```python
from build123d import *

# Parameters (mm, degrees)
SKETCH1_W      = 203.2
SKETCH1_H      = 101.6
EXTRUDE1_DEPTH = 50.8
EXTRUDE2_DEPTH = 16.51
SKETCH20_W     = 203.2
SKETCH20_H     = 50.8
EXTRUDE3_DEPTH = 1270


with BuildPart() as part:
    # Sketch1 → Extrude1 (new body)
    with BuildSketch(Plane.XY):
        with Locations((101.6, 50.8)):
            Rectangle(SKETCH1_W, SKETCH1_H)
    extrude(amount=EXTRUDE1_DEPTH)

    # Sketch6 → Extrude2 (add)
    with BuildSketch(Plane.XY.offset(50.8)):
        with BuildLine():
            ThreePointArc((37.627484075, 52.10066287), (41.730641244, 51.143940803), (45.529464649, 52.96607049))
            Line((45.529464649, 52.96607049), (64.421207315, 71.857813157))
            ThreePointArc((64.421207315, 71.857813157), (66.159065786, 75.109117673), (65.797714286, 78.777981013))
            Line((65.797714286, 78.777981013), (63.063921217, 85.377941317))
            Line((63.063921217, 85.377941317), (69.784164904, 91.197771623))
            Line((69.784164904, 91.197771623), (72.499996333, 84.641174554))
            Line((72.499996333, 84.641174554), (79.539958371, 87.557222308))
            Line((79.539958371, 87.557222308), (81.969998167, 81.690587277))
            Line((81.969998167, 81.690587277), (74.930036129, 78.774539522))
            Line((74.930036129, 78.774539522), (77.56029225, 72.424539522))
            Line((77.56029225, 72.424539522), (43.43531899, 38.299566262))
            Line((43.43531899, 38.299566262), (34.866461901, 43.758530283))
            Line((34.866461901, 43.758530283), (37.302310042, 45.218374053))
            Line((37.302310042, 45.218374053), (31.946774361, 48.630226566))
            Line((31.946774361, 48.630226566), (31.653140492, 45.805641791))
            Line((31.653140492, 45.805641791), (23.4233337, 51.04860695))
            Line((23.4233337, 51.04860695), (30.143577387, 56.868437256))
            Line((30.143577387, 56.868437256), (37.627484075, 52.10066287))
        make_face()
        Polygon((31.946774361, 48.630226566), (31.653140492, 45.805641791), (27.558917476, 39.378998974), (30.772238885, 37.331887466), (34.866461901, 43.758530283), (37.302310042, 45.218374053), align=None)
    extrude(amount=EXTRUDE2_DEPTH)

    # Sketch20 → Extrude3 (cut)
    with BuildSketch(Plane.XZ):
        with Locations((101.6, 25.4)):
            Rectangle(SKETCH20_W, SKETCH20_H)
    extrude(amount=-EXTRUDE3_DEPTH, mode=Mode.SUBTRACT)


solid = part.part
```
Part model, mm, in its own coordinate system. A direction names the side the tool comes from. Round coordinates to 2 decimals unless told otherwise and drop trailing zeros. Loops run counter-clockwise (first coordinate to the right, second up) from the corner with the lowest first, then second, coordinate; pieces in that order, holes last. Notation, with made-up numbers: (66, 20.5) -> (73, 20.5) arc R16 cw to (73, 38.5) -> close; hole circle Ø11 at (0.25, 66). An arc over 180 degrees is marked (long way). Use a Markdown table: item, result.
1) Cut at A-A, the plane x = 29. List the corners of the cut face in (y, z), and give its area (3 significant figures).
The answers:
| item | result |
|---|---|
| outline | (38.46, 50.8) -> (41.64, 50.8) -> (41.64, 67.31) -> (38.46, 67.31) -> close; (47.5, 50.8) -> (55.88, 50.8) -> (55.88, 67.31) -> (47.5, 67.31) -> close |
| area | 191 mm2 |
2) Cut at D-D, the plane x = 69. List the corners of the cut face in (y, z), and give its area (3 significant figures).
The answers:
| item | result |
|---|---|
| outline | (63.86, 50.8) -> (90.52, 50.8) -> (90.52, 67.31) -> (63.86, 67.31) -> close |
| area | 440 mm2 |
3) Cut at B-B, the plane z = 64.5. List the corners of the cut face in (x, y), and give its area (3 significant figures).
The answers:
| item | result |
|---|---|
| outline | (23.42, 51.05) -> (31.65, 45.81) -> (27.56, 39.38) -> (30.77, 37.33) -> (34.87, 43.76) -> (43.44, 38.3) -> (77.56, 72.42) -> (74.93, 78.77) -> (81.97, 81.69) -> (79.54, 87.56) -> (72.5, 84.64) -> (69.78, 91.2) -> (63.06, 85.38) -> (65.8, 78.78) arc R6.35 cw to (64.42, 71.86) -> (45.53, 52.97) arc R6.35 cw to (37.63, 52.1) -> (30.14, 56.87) -> close |
| area | 755 mm2 |
4) Tool access for faces 5 (the flat face through (32.79, 40.5, 58.94)), 6 (the flat face through (76.23, 75.64, 58.94)), 7 (the flat face through (27.6, 48.39, 58.94)), 8 (the flat face through (26.74, 53.92, 58.94)), 9 (the flat face through (71.12, 87.97, 58.94)): list every direction of +Z, -Z, +X, -X, +Y, -Y with a clear straight run to the whole face (end or side of a thin tool).
The answers:
| item | result |
|---|---|
| face 5 | +Z, -Z, -Y |
| face 6 | +Z, -Z, +X |
| face 7 | +Z, -Z, -X |
| face 8 | +Z, -Z, -X, +Y |
| face 9 | +Z, -Z, +Y |
5) Probe line 1 (Y direction, x = 65.5, z = 66); line 2 (Y direction, x = 28, z = 59); line 3 (X direction, y = 87, z = 56). List the from-to ranges inside material, lowest first. Write a range as [from, to].
The answers:
| item | result |
|---|---|
| line 1 | y = [60.36, 73.3], [79.5, 87.49] |
| line 2 | y = [39.1, 40.07], [48.13, 55.01] |
| line 3 | x = [64.94, 71.52], [78.19, 79.77] |
6) Cut at C-C, the plane y = 86.5. List the corners of the cut face in (x, z), and give its area (3 significant figures).
The answers:
| item | result |
|---|---|
| outline | (64.36, 50.8) -> (71.73, 50.8) -> (71.73, 67.31) -> (64.36, 67.31) -> close; (76.99, 50.8) -> (79.98, 50.8) -> (79.98, 67.31) -> (76.99, 67.31) -> close |
| area | 171 mm2 |
7) Pull direction X, two halves, no side cores. Call faces 1 (the flat face through (75.97, 86.08, 58.94)), 2 (the flat face through (80.74, 84.66, 58.94)), 3 (the flat face through (55, 62, 50.8)), 4 (the flat face through (29.14, 38.37, 58.94)): pulls with the +X half, pulls with the -X half, needs draft (parallel to the pull), parting line crosses it, or undercut.
The answers:
| item | result |
|---|---|
| face 1 | undercut |
| face 2 | pulls with the +X half |
| face 3 | needs draft |
| face 4 | pulls with the -X half |
8) Drop flat-ended pins along their axis: pin 1 Ø6 at (y, z) = (61, 62.5) entering from +X; pin 2 Ø3 at (y, z) = (44.5, 55) entering from -X; pin 3 Ø8 at (x, z) = (66, 58.5) entering from -Y. Give the stop position or say it passes through.
The answers:
| item | result |
|---|---|
| pin 1 | stops at x = 69.14 |
| pin 2 | stops at x = 29.87 |
| pin 3 | stops at y = 56.86 |
